from build123d import *

# Parameters (mm, degrees)
ESQUISSE1_R             = 15
BOSS_EXTRU_1_DEPTH      = 75
ENL_V_START             = -55
ESQUISSE2_R             = 15
ESQUISSE2_R_2           = 12.5
ENL_V_MAT_EXTRU_1_DEPTH = 55
CHANFREIN4_SIZE         = 0.2
CHANFREIN5_SIZE         = 0.2
ENL_V_MAT_EXTRU_2_DEPTH = 3


with BuildPart() as part:
    # Esquisse1 → Boss.-Extru.1 (new body)
    with BuildSketch(Plane(origin=(0, 0, 0), x_dir=(1, 0, 0), z_dir=(0, 1, 0))):
        with Locations(Location((0, 0, 0), (0, 0, 270))):
            Circle(ESQUISSE1_R)
    extrude(amount=BOSS_EXTRU_1_DEPTH)

    # Esquisse2 → Enlèv. mat.-Extru.1 (cut)
    with BuildSketch(Plane(origin=(0, 75, 0), x_dir=(1, 0, 0), z_dir=(0, 1, 0)).offset(ENL_V_START)):
        with Locations(Location((0, 0, 0), (0, 0, 270))):
            Circle(ESQUISSE2_R)
        with Locations(Location((0, 0, 0), (0, 0, 270))):
            Circle(ESQUISSE2_R_2, mode=Mode.SUBTRACT)
    extrude(amount=ENL_V_MAT_EXTRU_1_DEPTH, mode=Mode.SUBTRACT)

    # Chanfrein4
    chanfrein4_edges = [part.edges().sort_by_distance(p)[0] for p in [
        (0, 20, -15),
    ]]
    chamfer(chanfrein4_edges, length=CHANFREIN4_SIZE)

    # Chanfrein5
    chanfrein5_edges = [part.edges().sort_by_distance(p)[0] for p in [
        (0, 75, -12.5),
    ]]
    chamfer(chanfrein5_edges, length=CHANFREIN5_SIZE)

    # Esquisse3 → Enlèv. mat.-Extru.2 (cut)
    with BuildSketch(Plane(origin=(0, 0, -12.5), x_dir=(-1, 0, 0), z_dir=(0, 0, -1))):
        with BuildLine():
            Line((3.25, 70), (3.25, 45))
            ThreePointArc((3.25, 45), (0, 41.75), (-3.25, 45))
            Line((-3.25, 45), (-3.25, 70))
            ThreePointArc((-3.25, 70), (0, 73.25), (3.25, 70))
        make_face()
    extrude(amount=-ENL_V_MAT_EXTRU_2_DEPTH, mode=Mode.SUBTRACT)


solid = part.part
Work out the finished part from the listing and answer in its coordinate system (mm). A direction names the side the tool comes from. Coordinates: 2 decimals unless noted, no trailing zeros. Write each loop counter-clockwise with the first axis right and the second up, starting at its lowest first coordinate (ties: lowest second). Pieces come first, ordered by that corner, then holes. Notation, with made-up numbers: M -26,9 L 20,9 A12 cw 20,17 Z; hole C 40,31.25 d6. An arc over 180 degrees is marked long. Use one line per item in the form item = value. Start each with the question number.
1. The part is cut by section D-D (y = 17). Give the vertices of the cut face in (x, z), plus the area to 3 significant figures.
2. A tool of negligible diameter and unlimited length cuts with its end or side. For faces 1 (the face through (-0.07, 41.75, -11.02)), 2 (the face through (0, 75, 0)), 3 (the face through (-8, 20, -10)), from which of +Z, -Z, +X, -X, +Y, -Y can it reach the whole face along a straight path? Write none if from no direction.
3. The part is cut by section B-B (z = 0). Give the vertices of the cut face in (x, y).
4. Straight lines are drawn through the part: probe 1 along Y at (x, z) = (-1.5, -11.25); probe 2 along X at (y, z) = (59.5, -9.75); probe 3 along X at (y, z) = (4.5, -0.5). For each, find the intervals that lie inside material, in ascending order. Write a range as from..to.
5. Each of these flat-tipped pins is pushed along its axis until it touches: P1, Ø5, axis at x = 8.5, y = 64, coming from the -Z side; P2, Ø6, axis at x = -1.5, y = 59.5, coming from the +Z side; P3, Ø2, axis at x = 2, y = 27, coming from the -Z side. Where does it stop, or does it pass through?
6. The part is cut by section A-A (x = 0). Give the vertices of the cut face in (y, z).
7. The part is cut by section C-C (y = 57). Give the vertices of the cut face in (x, z).
8. The mould has two halves that part along X. Classify faces 4 (the face through (0, 0, 0)), 5 (the face through (3.755, 47.016, 11.923)), 6 (the face through (0.07, 73.25, -11.02)): released by +X, released by -X, zero draft, split by the parting line, or undercut.
Evaluation:
q1.outline = C 0,0 d30
q1.area = 707 mm^2
q2.face_1 = -Z
q2.face_2 = +Z, -Z, +X, -X, +Y
q2.face_3 = +Y
q3.outline = M -15,0 L 15,0 L 15,19.8 L 14.8,20 L 12.5,20 L 12.5,74.8 L 12.3,75 L -12.3,75 L -12.5,74.8 L -12.5,20 L -14.8,20 L -15,19.8 Z
q4.probe_1 = 0..42.12, 72.88..75
q4.probe_2 = -7.82..-3.25, 3.25..7.82
q4.probe_3 = -14.99..14.99
q5.P1 = -10.97
q5.P2 = 12.5
q5.P3 = -12.46
q6.outline = M 0,-15 L 19.8,-15 L 20,-14.8 L 20,-12.5 L 41.75,-12.5 L 41.75,-9.5 L 73.25,-9.5 L 73.25,-12.5 L 74.8,-12.5 L 75,-12.3 L 75,12.3 L 74.8,12.5 L 20,12.5 L 20,14.8 L 19.8,15 L 0,15 Z
q7.outline = M -3.25,-12.07 L -3.25,-9.5 L 3.25,-9.5 L 3.25,-12.07 A12.5 ccw long Z
q8.face_4 = zero draft
q8.face_5 = split by the parting line
q8.face_6 = undercut
